Geometry: final body of the model. Coordinates: model frame, mm. Face numbers are marked on the shaded views. A direction names the side the tool comes from. Give positions to 0.01 mm unless a question says otherwise; leave off trailing zeros. Order: outer loops, then holes, each group sorted by start corner. A loop starts at its lowest first (then second) coordinate and runs counter-clockwise, first axis right, second up. Notation, with made-up numbers: (9.5, 52) - (65.5, 52) arc R12 ccw to (65.5, 75) - close; hole circle Ø3 at (36, 24.25). An arc over 180 degrees is marked (long way). Use one line per item in the form item = value.
from build123d import *

# Parameters (mm, degrees)
CYLINDER003_R     = 3.6
CYLINDER003_DEPTH = 18
CYLINDER002_R     = 3.6
CYLINDER002_DEPTH = 18
CYLINDER001_R     = 3.6
CYLINDER001_DEPTH = 18
CYLINDER_R        = 3.6
CYLINDER_DEPTH    = 18
SKETCH_W          = 182
SKETCH_H          = 100
SKETCH_R          = 1.6
EXTRUDE001_DEPTH  = 17


with BuildPart() as zylinder003:
    # Cylinder003 → Cylinder003 (new body)
    with BuildSketch(Plane(origin=(86, -45, -14), x_dir=(1, 0, 0), z_dir=(0, 0, 1))):
        Circle(CYLINDER003_R)
    extrude(amount=CYLINDER003_DEPTH)


with BuildPart() as zylinder002:
    # Cylinder002 → Cylinder002 (new body)
    with BuildSketch(Plane(origin=(86, 45, -14), x_dir=(1, 0, 0), z_dir=(0, 0, 1))):
        Circle(CYLINDER002_R)
    extrude(amount=CYLINDER002_DEPTH)


with BuildPart() as zylinder001:
    # Cylinder001 → Cylinder001 (new body)
    with BuildSketch(Plane(origin=(-86, 45, -14), x_dir=(1, 0, 0), z_dir=(0, 0, 1))):
        Circle(CYLINDER001_R)
    extrude(amount=CYLINDER001_DEPTH)


with BuildPart() as fusion:
    # Cylinder → Cylinder (new body)
    with BuildSketch(Plane(origin=(-86, -45, -14), x_dir=(1, 0, 0), z_dir=(0, 0, 1))):
        Circle(CYLINDER_R)
    extrude(amount=CYLINDER_DEPTH)

    # Fusion: union Zylinder003, Zylinder002, Zylinder001
    add(zylinder003.part)
    add(zylinder002.part)
    add(zylinder001.part)


with BuildPart() as cut_aussen:
    # Sketch → Extrude001 (new body)
    with BuildSketch(Plane.XY):
        Rectangle(SKETCH_W, SKETCH_H)
        with Locations((-86, 45)):
            Circle(SKETCH_R, mode=Mode.SUBTRACT)
        with Locations((86, 45)):
            Circle(SKETCH_R, mode=Mode.SUBTRACT)
        with Locations((86, -45)):
            Circle(SKETCH_R, mode=Mode.SUBTRACT)
        with Locations((-86, -45)):
            Circle(SKETCH_R, mode=Mode.SUBTRACT)
        with BuildLine():
            Line((-84.520135, 48.5), (84.520135, 48.5))
            ThreePointArc((84.520135, 48.5), (82.986386, 42.685236), (89, 42.667619))
            Line((89, 42.667619), (89, -42.667619))
            ThreePointArc((89, -42.667619), (82.986386, -42.685236), (84.520135, -48.5))
            Line((84.520135, -48.5), (-84.520135, -48.5))
            ThreePointArc((-84.520135, -48.5), (-82.986386, -42.685236), (-89, -42.667619))
            Line((-89, -42.667619), (-89, 42.667619))
            ThreePointArc((-89, 42.667619), (-82.986386, 42.685236), (-84.520135, 48.5))
        make_face(mode=Mode.SUBTRACT)
    extrude(amount=-EXTRUDE001_DEPTH)

    # Cut006: cut Fusion
    add(fusion.part, mode=Mode.SUBTRACT)


solid = cut_aussen.part
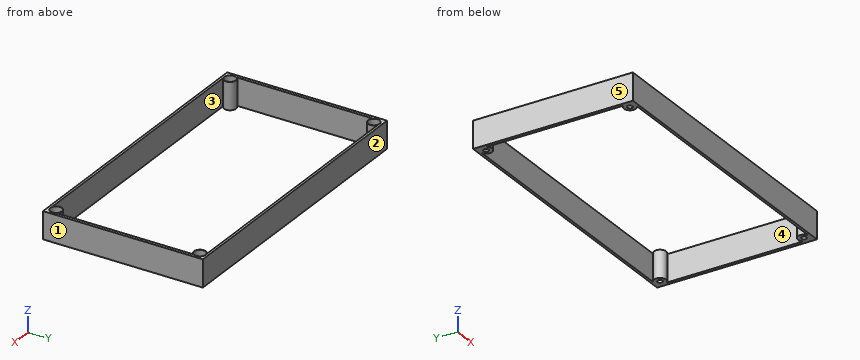
(1) Cut plane A-A on x = -69. Output: boundary loops of the cut face in (y, z), plus the area to 3 significant figures.
Computed values:
outline = (-50, -17) - (-48.5, -17) - (-48.5, 0) - (-50, 0) - close; (48.5, -17) - (50, -17) - (50, 0) - (48.5, 0) - close
area = 51.0 mm²
(2) Pull-direction query (X, two-part tool) for the marked faces 1, 2 and 3; classes: released by +X, released by -X, zero draft, split by the parting line, or undercut.
Computed values:
face_1 = released by +X
face_2 = zero draft
face_3 = undercut
(3) Cut plane B-B on y = 11.5. Output: boundary loops of the cut face in (x, z).
Computed values:
outline = (-91, -17) - (-89, -17) - (-89, 0) - (-91, 0) - close; (89, -17) - (91, -17) - (91, 0) - (89, 0) - close
(4) Contact query for flat-ended pins moving along their axis: pin 1 Ø3.5 at (x, y) = (86, 45) entering from +Z; pin 2 Ø3 at (x, y) = (-86, 45) entering from +Z. Output: stop coordinate, or through.
Computed values:
pin_1 = -14
pin_2 = through
(5) Reachability of the marked faces 4 and 5 from +Z, -Z, +X, -X, +Y, -Y: full face, straight path, thin tool, end or side. Return the list, or none.
Computed values:
face_4 = +Z, -Z
face_5 = +Z, -Z, -X, +Y, -Y
(6) Cut plane C-C on z = -3.25. Output: boundary loops of the cut face in (x, y).
Computed values:
outline = (-91, -50) - (91, -50) - (91, 50) - (-91, 50) - close; hole circle Ø7.2 at (-86, -45); hole circle Ø7.2 at (-86, 45); hole (-89, -42.67) arc R3.8 cw (long way) to (-84.52, -48.5) - (84.52, -48.5) arc R3.8 cw (long way) to (89, -42.67) - (89, 42.67) arc R3.8 cw (long way) to (84.52, 48.5) - (-84.52, 48.5) arc R3.8 cw (long way) to (-89, 42.67) - close; hole circle Ø7.2 at (86, -45); hole circle Ø7.2 at (86, 45)
(7) Ray query, line 1 along Y through (x, z) = (-86, -4.75); line 2 along X through (y, z) = (-45, -4.25); line 3 along Y through (x, z) = (-86, -14.55). Return the intervals inside material, ascending.
Computed values:
line_1 = -50 to -48.6, -41.4 to -41.2, 41.2 to 41.4, 48.6 to 50
line_2 = -91 to -89.6, -82.4 to -82.2, 82.2 to 82.4, 89.6 to 91
line_3 = -50 to -46.6, -43.4 to -41.2, 41.2 to 43.4, 46.6 to 50
